Design review of the part built by this model. Coordinates are the model's own, in mm. A direction names the side the tool comes from. Round coordinates to 2 decimals unless told otherwise and drop trailing zeros. Order: outer loops, then holes, each group sorted by start corner. A loop starts at its lowest first (then second) coordinate and runs counter-clockwise, first axis right, second up. Notation, with made-up numbers: (-13.75, 38) - (39.25, 38) arc R19 ccw to (39.25, 63) - close; hole circle Ø1 at (-21, 47.5). An arc over 180 degrees is marked (long way). Write item = value, one per line.
from build123d import *

# Parameters (mm, degrees)
SKETCH1_W           = 100
SKETCH1_H           = 125
BOSS_EXTRUDE1_DEPTH = 40


with BuildPart() as part:
    # Sketch1 → Boss-Extrude1 (new body)
    with BuildSketch(Plane(origin=(0, 0, 0), x_dir=(1, 0, 0), z_dir=(0, 1, 0))):
        with BuildLine():
            ThreePointArc((-55, -24.644660941), (-30, -85), (30.355339059, -110))
            Line((30.355339059, -110), (55, -110))
            Line((55, -110), (55, 15))
            Line((55, 15), (55, 110))
            Line((55, 110), (-55, 110))
            Line((-55, 110), (-55, -24.644660941))
        make_face()
        with Locations((105, -47.5)):
            Rectangle(SKETCH1_W, SKETCH1_H)
        Polygon((155, 15), (155, -110), (265, -110), (265, 110), (155, 110), align=None)
    extrude(amount=BOSS_EXTRUDE1_DEPTH)


solid = part.part
Item 1: For faces 1 (the face through (211, 20, -110)), 2 (the face through (55, 20, -62)), list the 3-axis set-ups (+Z, -Z, +X, -X, +Y, -Y) from which the entire face can be reached by the end or side of a thin tool; tool diameter is ignored.
Data:
face_1 = -Z, +X, -X, +Y, -Y
face_2 = -Z, +Y, -Y
Item 2: For line 1 along X through (y, z) = (38.5, -98); line 2 along Z through (x, y) = (62, 28.5); line 3 along X through (y, z) = (32, 88), list the stretches that pass through material, from the lowest coordinate up. Write a range as [from, to].
Data:
line_1 = [-55, 55], [155, 265]
line_2 = [-15, 110]
line_3 = [-26.84, 265]
Item 3: The part is to be moulded in two halves that separate along X. For faces 3 (the face through (155, 20, -63)), 4 (the face through (104, 20, -15)), 5 (the face through (103, 0, -2)), 6 (the face through (265, 20, 2)), say which applies: +X half, -X half, draft (parallel to the pull), parting line (faces both ways), or undercut.
Data:
face_3 = undercut
face_4 = undercut
face_5 = draft
face_6 = +X half
Item 4: Take a section at B-B, the plane y = 15.5. State the section outline as (x, z) points.
Data:
outline = (-55, -110) - (55, -110) - (55, -15) - (155, -15) - (155, -110) - (265, -110) - (265, 110) - (30.36, 110) arc R85.36 ccw to (-55, 24.64) - close
Item 5: Take a section at C-C, the plane z = 73. State the section outline as (x, y) points.
Data:
outline = (-39.98, 0) - (265, 0) - (265, 40) - (-39.98, 40) - close
Item 6: Take a section at A-A, the plane z = -78.5. State the section outline as (x, y) points.
Data:
outline = (-55, 0) - (55, 0) - (55, 40) - (-55, 40) - close; (155, 0) - (265, 0) - (265, 40) - (155, 40) - close
Item 7: Insertion check: P1, Ø10, axis at x = 107, y = 14, coming from the -Z side. The pin has a flat end and moves straight along its axis. Give the tip position at first contact, or say it passes through.
Data:
P1 = -15
